from build123d import *

# Parameters (mm, degrees)
SKETCH1_R           = 40
BOSS_EXTRUDE1_DEPTH = 100
SKETCH3_R           = 10
CUT_EXTRUDE1_DEPTH  = 115.891252931


with BuildPart() as part:
    # Sketch1 → Boss-Extrude1 (new body)
    with BuildSketch(Plane(origin=(0, 0, 0), x_dir=(0, 0, -1), z_dir=(1, 0, 0))):
        Circle(SKETCH1_R)
    extrude(amount=BOSS_EXTRUDE1_DEPTH)

    # Sketch2 → Cut-Revolve1 (revolve, cut)
    with BuildSketch(Plane(origin=(0, 0, 0), x_dir=(1, 0, 0), z_dir=(0, 1, 0)), mode=Mode.PRIVATE) as cut_revolve1_sk:
        Polygon((9.736892583, 40), (30.975149321, 11.906444473), (69.024850679, 11.906444473), (90.263107417, 40), align=None)
    revolve(cut_revolve1_sk.sketch.rotate(Axis((0, 0, 0), (1, 0, 0)), 180), axis=Axis((0, 0, 0), (1, 0, 0)), mode=Mode.SUBTRACT)

    # Sketch3 → Cut-Extrude1 (cut, through all)
    with BuildSketch(Plane.ZY):
        Circle(SKETCH3_R)
    extrude(amount=-CUT_EXTRUDE1_DEPTH, mode=Mode.SUBTRACT)


solid = part.part
Build history of the part. All positions in model axes, mm. A direction names the side the tool comes from. Coordinates: 2 decimals unless noted, no trailing zeros. Write each loop counter-clockwise with the first axis right and the second up, starting at its lowest first coordinate (ties: lowest second). Pieces come first, ordered by that corner, then holes.
(1) Pin check, flat tips, straight feed: pin 1 Ø18 at (y, z) = (0, 0) entering from +X; pin 2 Ø1.5 at (x, z) = (76, -2.5) entering from +Y; pin 3 Ø6 at (x, y) = (32, -3) entering from +Z; pin 4 Ø3 at (x, z) = (79, -17) entering from -Y. Stop position of each tip, or through.
(2) Drill centre lines: line 1 (Y direction, x = 52, z = 0); line 2 (X direction, y = 8, z = 9); line 3 (X direction, y = 5, z = 20). Where is each one in solid material? Low to high.
(3) Cut at D-D on x = 14. List the corners of the cut face in (y, z).
(4) Mould opens along Y. For faces 1 (the cylindrical face through (49.3, -9.76, -2.17)), 2 (the cylindrical face through (4.8, -39.05, 8.67)), 3 (the flat face through (0, -8, -8)) say: pulls with the +Y half, pulls with the -Y half, needs draft (parallel to the pull), parting line crosses it, or undercut.
(5) 3-axis set-ups, long thin cutter, end or side, ignore diameter. For faces 4 (the conical face through (70.35, -4.1, 13.03)), 5 (the cylindrical face through (95.06, -39.05, 8.67)): which of +Z, -Z, +X, -X, +Y, -Y reach the whole face in a straight line?
(6) Cut at C-C on x = 61.5. List the corners of the cut face in (y, z).
(7) Cut at A-A on y = 0. List the corners of the cut face in (x, z), and give its area (3 significant figures).
Working result:
1. pin 1: passes through
1. pin 2: stops at y = 21.99
1. pin 3: stops at z = 14.25
1. pin 4: stops at y = -21.35
2. line 1: y = -11.91 to -10, 10 to 11.91
2. line 2: x = 0 to 30.87, 69.13 to 100
2. line 3: x = 0 to 24.39, 75.61 to 100
3. outline: circle Ø68.72 at (0, 0); hole circle Ø20 at (0, 0)
4. face 1: undercut
4. face 2: parting line crosses it
4. face 3: needs draft
5. face 4: none
5. face 5: +X, -X
6. outline: circle Ø23.81 at (0, 0); hole circle Ø20 at (0, 0)
7. outline: (0, -40) - (9.74, -40) - (30.98, -11.91) - (69.02, -11.91) - (90.26, -40) - (100, -40) - (100, -10) - (0, -10) - close; (0, 10) - (100, 10) - (100, 40) - (90.26, 40) - (69.02, 11.91) - (30.98, 11.91) - (9.74, 40) - (0, 40) - close
7. area: 2,670 mm2
